For this review, take the finished solid that the model builds, in its own axes (mm). A direction names the side the tool comes from. Round coordinates to 2 decimals unless told otherwise and drop trailing zeros. Order: outer loops, then holes, each group sorted by start corner. A loop starts at its lowest first (then second) coordinate and runs counter-clockwise, first axis right, second up. Notation, with made-up numbers: (51.5, -23) - (66.5, -23) arc R16 cw to (66.5, -18) - close; hole circle Ø9 at (42.25, 75.25). An arc over 180 degrees is marked (long way). Write each question's results on one line, items separated by ' | '. Start each with the question number.
(1) Draft analysis for pull direction X (two halves, no side actions). For faces 4 (the flat face through (2.96, 2.96, 5.22)), 5 (the flat face through (-3.042, 2.958, 5.172)), 6 (the cylindrical face through (3, -6, 0)), state which applies: pulls with the +X half, pulls with the -X half, needs draft (parallel to the pull), parting line crosses it, or undercut.
(2) Take a section at D-D, the plane x = 0.75. Give the boundary of the cut face in (y, z).
(3) Take a section at C-C, the plane x = -4. Give the boundary of the cut face in (y, z).
(4) Insertion check: pin 1 Ø8 at (y, z) = (-8, -3) entering from +X; pin 2 Ø1.5 at (x, y) = (1.5, -2) entering from -Z; pin 3 Ø4 at (x, y) = (-4.5, -3) entering from -Z. Each pin has a flat end and moves straight along its axis. Give the tip position at first contact, or say it passes through.
(5) For faces 1 (the cylindrical face through (-4, -5, 0)), 2 (the cylindrical face through (5.453, -5.916, 0.716)), 3 (the flat face through (-6, 3, 0)), list the 3-axis set-ups (+Z, -Z, +X, -X, +Y, -Y) from which the entire face can be reached by the end or side of a thin tool; tool diameter is ignored.
(6) Take a section at B-B, the plane y = 0.5. Give the boundary of the cut face in (x, z).
(7) For L1, parallel to Y at x = -4.7, z = 0; L2, parallel to Y at x = 5, z = -4; L3, parallel to X at y = -4.25, z = 0, list the stretches that pass through material, from the lowest coordinate up. Write a range as from..to.
(8) Take a section at A-A, the plane z = 0. Give the boundary of the cut face in (x, y), plus the area to 3 significant figures.
```python
from build123d import *

# Parameters (mm, degrees)
EXTRUDE_1_DEPTH     = 6
SKETCH_2_R          = 5.5
EXTRUDE_2_DEPTH     = 12
SKETCH_3_R          = 2
CUT_EXTRUDE_1_DEPTH = 12
SKETCH_4_R          = 3
CUT_EXTRUDE_2_DEPTH = 12


with BuildPart() as part:
    # 草图1 → 凸台-拉伸1 (new body)
    with BuildSketch(Plane(origin=(0, 0, 0), x_dir=(1, 0, 0), z_dir=(0, 1, 0))):
        Polygon((0, 6.92820323), (-6, 3.464101615), (-6, -3.464101615), (0, -6.92820323), (6, -3.464101615), (6, 3.464101615), align=None)
    extrude(amount=EXTRUDE_1_DEPTH)

    # 草图2 → 凸台-拉伸2 (add)
    with BuildSketch(Plane.XZ):
        with Locations(Location((0, 0, 0), (0, 0, 270))):
            Circle(SKETCH_2_R)
    extrude(amount=EXTRUDE_2_DEPTH)

    # 草图3 → 切除-拉伸1 (cut)
    with BuildSketch(Plane(origin=(0, 0, 0), x_dir=(0, 0, -1), z_dir=(1, 0, 0))):
        with Locations((0, -7)):
            Circle(SKETCH_3_R)
    extrude(amount=-CUT_EXTRUDE_1_DEPTH, mode=Mode.SUBTRACT)

    # 草图4 → 切除-拉伸2 (cut)
    with BuildSketch(Plane.XZ.offset(12)):
        with Locations(Location((0, 0, 0), (0, 0, 270))):
            Circle(SKETCH_4_R)
    extrude(amount=-CUT_EXTRUDE_2_DEPTH, mode=Mode.SUBTRACT)


solid = part.part
```
Results below:
1) face 4: pulls with the +X half | face 5: pulls with the -X half | face 6: undercut
2) outline: (-12, -5.45) - (0, -5.45) - (0, -6.5) - (6, -6.5) - (6, 6.5) - (0, 6.5) - (0, 5.45) - (-12, 5.45) - (-12, 2.9) - (0, 2.9) - (0, -2.9) - (-12, -2.9) - close
3) outline: (-12, -3.77) - (0, -3.77) - (0, -4.62) - (6, -4.62) - (6, 4.62) - (0, 4.62) - (0, 3.77) - (-12, 3.77) - close; hole circle Ø4 at (-7, 0)
4) pin 1: stops at x = 5.5 | pin 2: stops at z = -5.45 | pin 3: stops at z = -4.9
5) face 1: -X | face 2: -Y | face 3: +Z, -Z, -X, +Y, -Y
6) outline: (-6, -3.46) - (0, -6.93) - (6, -3.46) - (6, 3.46) - (0, 6.93) - (-6, 3.46) - close
7) L1: y = -12..-9, -5..6 | L2: y = 0..6 | L3: x = -5.5..-3, 3..5.5
8) outline: (-6, 0) - (-5.5, 0) - (-5.5, -5) - (-3, -5) - (-3, 0) - (3, 0) - (3, -12) - (5.5, -12) - (5.5, 0) - (6, 0) - (6, 6) - (-6, 6) - close; (-5.5, -12) - (-3, -12) - (-3, -9) - (-5.5, -9) - close | area: 122 mm^2
